```python
from build123d import *

# Parameters (mm, degrees)
F0_W      = 80
F0_H      = 60
F1_DEPTH  = 50
F2_R      = 20
F3_W      = 5
F3_H      = 10
F4_DEPTH  = 30
F6_W      = 50
F6_H      = 30
F7_DEPTH  = 40
F8_R      = 5
F9_DEPTH  = 10
F10_R     = 20
F11_DEPTH = 10
F12_SIZE2 = 5
F12_SIZE  = 10


with BuildPart() as f1:
    # F0 (on Top) → F1 (new body)
    with BuildSketch(Plane.XY):
        with Locations((40, 30)):
            Rectangle(F0_W, F0_H)
    extrude(amount=F1_DEPTH)

    # F2
    f2_edges = [f1.edges().sort_by_distance(p)[0] for p in [
        (80, 30, 50),
    ]]
    fillet(f2_edges, radius=F2_R)


with BuildPart() as f4:
    # F3 (on face) → F4 (new body)
    with BuildSketch(Plane.XZ):
        with Locations((2.5, 55)):
            Rectangle(F3_W, F3_H)
    extrude(amount=-F4_DEPTH)


with BuildPart() as f1_1:
    add(f1.part)

    # F5: union F4
    add(f4.part)

    # F6 (on face) → F7 (cut)
    with BuildSketch(Plane.XZ):
        with Locations((55, 15)):
            Rectangle(F6_W, F6_H)
    extrude(amount=-F7_DEPTH, mode=Mode.SUBTRACT)

    # F8 (on face) → F9 (cut)
    with BuildSketch(Plane.XZ.offset(-40)):
        with Locations((70, 15)):
            Circle(F8_R)
    extrude(amount=-F9_DEPTH, mode=Mode.SUBTRACT)

    # F10 (on face) → F11 (join)
    with BuildSketch(Plane.XY.offset(50)):
        with Locations((40, 30)):
            Circle(F10_R)
    extrude(amount=F11_DEPTH)

    # F12
    f12_edges = [f1_1.edges().sort_by_distance(p)[0] for p in [
        (20, 30, 60),
    ]]
    f12_side = f1_1.faces().sort_by_distance((40, 30, 60))[0]
    chamfer(f12_edges, length=F12_SIZE, length2=F12_SIZE2, reference=f12_side)


solid = f1_1.part
```
The listing builds one solid part. Answer for the finished solid, in the listing's coordinates (mm). A direction names the side the tool comes from. Round coordinates to 2 decimals unless told otherwise and drop trailing zeros. Order: outer loops, then holes, each group sorted by start corner. A loop starts at its lowest first (then second) coordinate and runs counter-clockwise, first axis right, second up. Notation, with made-up numbers: (86.5, 46) -> (106.5, 46) arc R12 cw to (106.5, 51) -> close; hole circle Ø8 at (68, -4). An arc over 180 degrees is marked (long way). Answer as CSV lines item,"result". Start each with the question number.
(1) The part is cut by section C-C (z = 15). Determine the outline of the cut face in (x, y), then the cut area to 3 significant figures.
(2) The part is cut by section D-D (z = 42). Determine the outline of the cut face in (x, y).
(3) The part is cut by section A-A (y = 5). Determine the outline of the cut face in (x, z), then the cut area to 3 significant figures.
(4) Find the intervals of material crossed by probe 1 along X at (y, z) = (5.5, 3); probe 2 along Z at (x, y) = (45, 24.5); probe 3 along Z at (x, y) = (70, 43), in increasing order. Write a range as from..to.
(5) A tool of negligible diameter and unlimited length cuts with its end or side. For faces 5 (the face through (5, 15, 55)), 6 (the face through (16, 30, 50)), 7 (the face through (30, 20, 15)), 8 (the face through (2, 30, 55)), 9 (the face through (2, 15, 60)), from which of +Z, -Z, +X, -X, +Y, -Y can it reach the whole face along a straight path? Write none if from no direction.
(6) Flat-ended cylindrical pins translate along their axes: pin 1 Ø20 at (x, y) = (54, 11.5) entering from -Z; pin 2 Ø1.5 at (x, z) = (68.5, 7) entering from -Y; pin 3 Ø4 at (y, z) = (39.5, 36) entering from +X; pin 4 Ø8 at (x, z) = (16, 42.5) entering from -Y. Find the tip coordinate at first contact, or state that the pin passes through.
(7) For a pull along Z with two mould halves and no side action, classify faces 1 (the face through (70, 50, 15)), 2 (the face through (0, 30, 30)), 3 (the face through (74.619, 44.93, 13.085)), 4 (the face through (55, 20, 30)) as +Z half, -Z half, draft (parallel to the pull), parting line (faces both ways), or undercut.
(8) The part is cut by section B-B (x = 40). Determine the outline of the cut face in (y, z).
Evaluation:
1,outline,"(0, 0) -> (30, 0) -> (30, 40) -> (65, 40) -> (65, 50) -> (75, 50) -> (75, 40) -> (80, 40) -> (80, 60) -> (0, 60) -> close"
1,area,"2,700 mm²"
2,outline,"(0, 0) -> (76, 0) -> (76, 60) -> (0, 60) -> close"
3,outline,"(0, 0) -> (30, 0) -> (30, 30) -> (80, 30) arc R20 ccw to (60, 50) -> (5, 50) -> (5, 60) -> (0, 60) -> close"
3,area,"2,460 mm²"
4,probe 1,"0..30"
4,probe 2,"30..60"
4,probe 3,"0..10, 20..47.32"
5,face 5,"+Z, +Y, -Y"
5,face 6,"+Z"
5,face 7,"-Z, +X, -Y"
5,face 8,"+Z, -X, +Y"
5,face 9,"+Z, +X, -X, +Y, -Y"
6,pin 1,"z = 30"
6,pin 2,"y = 40"
6,pin 3,"x = 79.6"
6,pin 4,"y = 0"
7,face 1,"undercut"
7,face 2,"draft"
7,face 3,"undercut"
7,face 4,"-Z half"
8,outline,"(0, 30) -> (40, 30) -> (40, 0) -> (60, 0) -> (60, 50) -> (50, 50) -> (50, 55) -> (40, 60) -> (20, 60) -> (10, 55) -> (10, 50) -> (0, 50) -> close"
